The listing builds one solid part. Answer for the finished solid, in the listing's coordinates (mm). A direction names the side the tool comes from. Round coordinates to 2 decimals unless told otherwise and drop trailing zeros. Loops run counter-clockwise (first coordinate to the right, second up) from the corner with the lowest first, then second, coordinate; pieces in that order, holes last. Notation, with made-up numbers: (57, -19) - (77, -19) arc R24 ccw to (77, -9) - close; hole circle Ø11 at (49, 35). An arc over 180 degrees is marked (long way). One line per question, with ' | ' between items. Start each with the question number.
from build123d import *

# Parameters (mm, degrees)
BOSS_EXTRUDE1_DEPTH = 6.35
CUT_EXTRUDE1_DEPTH  = 7.35
SKETCH3_R           = 2.1
CUT_EXTRUDE2_DEPTH  = 7.35
SKETCH4_R           = 2.1
CUT_EXTRUDE3_DEPTH  = 7.35
SKETCH5_R           = 4.85
CUT_EXTRUDE4_DEPTH  = 7.35


with BuildPart() as part:
    # Sketch1 → Boss-Extrude1 (new body)
    with BuildSketch(Plane.XY):
        Polygon((-89.75, 0), (89.75, 0), (89.75, 12), (84.75, 17), (84.75, 306), (89.75, 311), (89.75, 340), (-89.75, 340), (-89.75, 311), (-84.75, 306), (-84.75, 17), (-89.75, 12), align=None)
    extrude(amount=BOSS_EXTRUDE1_DEPTH)

    # Sketch2 → Cut-Extrude1 (cut, through all)
    with BuildSketch(Plane.XY.offset(6.35)):
        with BuildLine():
            Line((-49.5, 181.866529721), (49.5, 181.866529721))
            ThreePointArc((49.5, 181.866529721), (51.621320344, 180.987850064), (52.5, 178.866529721))
            Line((52.5, 178.866529721), (52.5, 57.132206767))
            ThreePointArc((52.5, 57.132206767), (51.621320344, 55.010886424), (49.5, 54.132206767))
            Line((49.5, 54.132206767), (-49.5, 54.132206767))
            ThreePointArc((-49.5, 54.132206767), (-51.621320344, 55.010886424), (-52.5, 57.132206767))
            Line((-52.5, 57.132206767), (-52.5, 178.866529721))
            ThreePointArc((-52.5, 178.866529721), (-51.621320344, 180.987850064), (-49.5, 181.866529721))
        make_face()
    extrude(amount=-CUT_EXTRUDE1_DEPTH, mode=Mode.SUBTRACT)

    # Sketch3 → Cut-Extrude2 (cut, through all)
    with BuildSketch(Plane.XY.offset(6.35)):
        with Locations((-64.5, 75.499368245)):
            Circle(SKETCH3_R)
        with Locations((-64.5, 90.499368245)):
            Circle(SKETCH3_R)
        with Locations((-64.5, 134.499368243)):
            Circle(SKETCH3_R)
        with Locations((-64.5, 119.499368243)):
            Circle(SKETCH3_R)
        with Locations((-64.5, 193.905249142)):
            Circle(SKETCH3_R)
        with Locations((64.5, 163.499368242)):
            Circle(SKETCH3_R)
        with Locations((64.5, 178.499368242)):
            Circle(SKETCH3_R)
        with Locations((71.501617277, 155.85352801)):
            Circle(SKETCH3_R)
        with Locations((71.501617277, 111.85352804)):
            Circle(SKETCH3_R)
    extrude(amount=-CUT_EXTRUDE2_DEPTH, mode=Mode.SUBTRACT)

    # Sketch4 → Cut-Extrude3 (cut, through all)
    with BuildSketch(Plane.XY.offset(6.35)):
        with Locations((-34, 332)):
            Circle(SKETCH4_R)
        with Locations((34, 332)):
            Circle(SKETCH4_R)
        with Locations((34, 284)):
            Circle(SKETCH4_R)
        with Locations((-34, 284)):
            Circle(SKETCH4_R)
        with Locations((-34, 8)):
            Circle(SKETCH4_R)
        with Locations((-34, 22.001)):
            Circle(SKETCH4_R)
        with Locations((34, 22.001)):
            Circle(SKETCH4_R)
        with Locations((34, 8)):
            Circle(SKETCH4_R)
    extrude(amount=-CUT_EXTRUDE3_DEPTH, mode=Mode.SUBTRACT)

    # Sketch5 → Cut-Extrude4 (cut, through all)
    with BuildSketch(Plane.XY.offset(6.35)):
        with Locations((0, 15.0005)):
            Circle(SKETCH5_R)
    extrude(amount=-CUT_EXTRUDE4_DEPTH, mode=Mode.SUBTRACT)


solid = part.part
(1) Determine the mould class of faces 1 (the flat face through (89.75, 325, 3)), 2 (the flat face through (-1, 0, 3)), 3 (the flat face through (52.5, 119, 3)) for opening direction Y: pulls with the +Y half, pulls with the -Y half, needs draft (parallel to the pull), parting line crosses it, or undercut.
(2) Find section A-A on x = -24. Write down the section's boundary in (y, z), plus the area to 3 significant figures.
(3) Each of these flat-tipped pins is pushed along its axis until it touches: P1, Ø1.9, axis at y = 111.5, z = 2, coming from the +X side; P2, Ø3.5, axis at x = 71.5, y = 111.85, coming from the -Z side; P3, Ø5.5, axis at x = -34, y = 22.001, coming from the +Z side; P4, Ø3, axis at y = 142, z = 2.5, coming from the -X side. Where does it stop, or does it pass through?
(4) A tool of negligible diameter and unlimited length cuts with its end or side. For faces 4 (the flat face through (-84.75, 164, 3)), 5 (the flat face through (84.75, 159, 3)), 6 (the flat face through (1, 54.132, 3)), from which of +Z, -Z, +X, -X, +Y, -Y can it reach the whole face along a straight path? Write none if from no direction.
(5) Find section C-C on y = 291.5. Write down the section's boundary in (x, z), plus the area to 3 significant figures.
(6) Consider L1, parallel to Y at x = 64.5, z = 1.5; L2, parallel to Y at x = -64.5, z = 2.5; L3, parallel to X at y = 332, z = 3.5. Determine where each line is inside the solid, lowest interval first.
(7) Find section D-D on z = 1.5. Count the separate pieces of the cut face and the enclosed holes in it, plus the area to 3 significant figures.
(8) Find section B-B on x = 0. Write down the section's boundary in (y, z).
Answer below:
1) face 1: needs draft | face 2: pulls with the -Y half | face 3: undercut
2) outline: (0, 0) - (54.13, 0) - (54.13, 6.35) - (0, 6.35) - close; (181.87, 0) - (340, 0) - (340, 6.35) - (181.87, 6.35) - close | area: 1,350 mm2
3) P1: x = 84.75 | P2: through | P3: z = 6.35 | P4: x = -84.75
4) face 4: +Z, -Z, -X | face 5: +Z, -Z, +X | face 6: +Z, -Z
5) outline: (-84.75, 0) - (84.75, 0) - (84.75, 6.35) - (-84.75, 6.35) - close | area: 1,080 mm2
6) L1: 0 to 161.4, 165.6 to 176.4, 180.6 to 340 | L2: 0 to 73.4, 77.6 to 88.4, 92.6 to 117.4, 121.6 to 132.4, 136.6 to 191.81, 196.01 to 340 | L3: -89.75 to -36.1, -31.9 to 31.9, 36.1 to 89.75
7) separate pieces: 1 | enclosed holes: 19 | area: 44,400 mm2
8) outline: (0, 0) - (10.15, 0) - (10.15, 6.35) - (0, 6.35) - close; (19.85, 0) - (54.13, 0) - (54.13, 6.35) - (19.85, 6.35) - close; (181.87, 0) - (340, 0) - (340, 6.35) - (181.87, 6.35) - close
